```python
from build123d import *

# Parameters (mm, degrees)
SKETCH_1_R          = 2.5
EXTRUDE_1_DEPTH     = 4
EXTRUDE_2_DEPTH     = 20.7
SKETCH_3_R          = 3
CUT_EXTRUDE_1_DEPTH = 6.7
CUT_EXTRUDE_2_DEPTH = 10


with BuildPart() as part:
    # Эскиз1 → Бобышка-Вытянуть1 (new body)
    with BuildSketch(Plane.XY):
        Polygon((0, 0), (108, 0), (108, 30), (55, 50), (55, 68), (0, 68), align=None)
        with Locations((21, 57)):
            Circle(SKETCH_1_R, mode=Mode.SUBTRACT)
        with Locations((49, 57)):
            Circle(SKETCH_1_R, mode=Mode.SUBTRACT)
        with Locations((21, 11)):
            Circle(SKETCH_1_R, mode=Mode.SUBTRACT)
        with Locations((49, 11)):
            Circle(SKETCH_1_R, mode=Mode.SUBTRACT)
        with Locations((88, 10)):
            Circle(SKETCH_1_R, mode=Mode.SUBTRACT)
        with Locations((88, 25)):
            Circle(SKETCH_1_R, mode=Mode.SUBTRACT)
    extrude(amount=EXTRUDE_1_DEPTH)

    # Эскиз2 → Бобышка-Вытянуть2 (add)
    with BuildSketch(Plane.XY.offset(4)):
        Polygon((108, 0), (104, 0), (104, 31.509433962), (108, 30), align=None)
    extrude(amount=-EXTRUDE_2_DEPTH)

    # Эскиз3 → Вырез-Вытянуть1 (cut)
    with BuildSketch(Plane(origin=(108, 0, 0), x_dir=(0, 0, -1), z_dir=(1, 0, 0))):
        with Locations((6, 10)):
            Circle(SKETCH_3_R)
    extrude(amount=-CUT_EXTRUDE_1_DEPTH, mode=Mode.SUBTRACT)

    # Эскиз4 → Вырез-Вытянуть2 (cut)
    with BuildSketch(Plane(origin=(0, 0, 0), x_dir=(-1, 0, 0), z_dir=(0, 0, -1))):
        Polygon((0, 68), (-15, 68), (-15, 48), (-15, 28), (-10, 28), (-10, 58), (0, 58), align=None)
    extrude(amount=-CUT_EXTRUDE_2_DEPTH, mode=Mode.SUBTRACT)


solid = part.part
```
Part model, mm, in its own coordinate system. A direction names the side the tool comes from. Round coordinates to 2 decimals unless told otherwise and drop trailing zeros. Write each loop counter-clockwise with the first axis right and the second up, starting at its lowest first coordinate (ties: lowest second). Pieces come first, ordered by that corner, then holes. Notation, with made-up numbers: M 74,68.25 L 82,68.25 A28 ccw 82,103.25 Z; hole C 24.25,6 d1. An arc over 180 degrees is marked long. Answer as CSV lines item,"result". Start each with the question number.
1) Band-saw the part on C-C (y = 41). List the corners of the cut face in (x, z).
2) Which spindle directions (+Z, -Z, +X, -X, +Y, -Y) get a long thin tool onto all of the face, cutting with end or side? Do faces 1 (the face through (40, 27, 0)), 2 (the face through (55, 59, 2)), 3 (the face through (13, 28, 2)), 4 (the face through (5, 58, 2)). Say none if no direction does.
3) Band-saw the part on B-B (y = 53). List the corners of the cut face in (x, z).
4) Drop flat-ended pins along their axis: pin 1 (2 mm diameter, centred on x = 13.5, z = 1.5, fed in from +Y); pin 2 (6 mm diameter, centred on x = 21, y = 11, fed in from -Z); pin 3 (3 mm diameter, centred on x = 5.5, z = 1.5, fed in from +Y). Give the stop position or say it passes through.
5) Band-saw the part on A-A (x = 49). List the corners of the cut face in (y, z), then the cut area to 3 significant figures.
6) Mould opens along X. For faces 5 (the face through (106.03, 8.85, -8.77)), 6 (the face through (104, 16, -8)), 7 (the face through (10, 43, 2)) say: +X half, -X half, draft (parallel to the pull), parting line (faces both ways), or undercut.
7) Drill centre lines: L1, parallel to Y at x = 21, z = 0.9; L2, parallel to Y at x = 50.5, z = 0.5; L3, parallel to Z at x = 57.5, y = 29.5. Where is each one in solid material? Low to high.
8) Band-saw the part on D-D (x = 88). List the corners of the cut face in (y, z), then the cut area to 3 significant figures.
Worked out:
1,outline,"M 0,0 L 10,0 L 10,4 L 0,4 Z; M 15,0 L 78.85,0 L 78.85,4 L 15,4 Z"
2,face 1,"-Z, -X, +Y, -Y"
2,face 2,"+Z, -Z, +X, +Y"
2,face 3,"+Z, -Z, +Y"
2,face 4,"+Z, -Z, -X, +Y"
3,outline,"M 0,0 L 10,0 L 10,4 L 0,4 Z; M 15,0 L 55,0 L 55,4 L 15,4 Z"
4,pin 1,"y = 28"
4,pin 2,"z = 0"
4,pin 3,"y = 58"
5,outline,"M 0,0 L 8.5,0 L 8.5,4 L 0,4 Z; M 13.5,0 L 54.5,0 L 54.5,4 L 13.5,4 Z; M 59.5,0 L 68,0 L 68,4 L 59.5,4 Z"
5,area,"232 mm²"
6,face 5,"draft"
6,face 6,"-X half"
6,face 7,"undercut"
7,L1,"0 to 8.5, 13.5 to 54.5, 59.5 to 68"
7,L2,"0 to 9, 13 to 55, 59 to 68"
7,L3,"0 to 4"
8,outline,"M 0,0 L 7.5,0 L 7.5,4 L 0,4 Z; M 12.5,0 L 22.5,0 L 22.5,4 L 12.5,4 Z; M 27.5,0 L 37.55,0 L 37.55,4 L 27.5,4 Z"
8,area,"110 mm²"
